Autodesk Inventor part; units mm, degrees
ref_plane "YZ Plane" through (0, 0, 0) normal (1, 0, 0) x (0, 1, 0)
ref_plane "XZ Plane" through (0, 0, 0) normal (0, 1, 0) x (-1, 0, 0)
ref_plane "XY Plane" through (0, 0, 0) normal (0, 0, 1) x (1, 0, 0)
sketch "草图1" plane through (0, 0, 0) normal (0, 1, 0) x (-1, 0, 0)
  circle A0 centre (-2.0908, 11.2121) radius 1.25
  line L0 (-5.7974, 4.2121) -> (1.6092, -1.1691) construction
  circle A1 centre (-11.3094, -1.4762) radius 1.25
  line L1 (0.7195, 14.068) -> (0.7195, -0.5227)
  line L2 (-4.7634, 3.4608) -> (-4.7634, 14.068)
  line L3 (-4.7634, 14.068) -> (0.7195, 14.068)
  line L4 (-13.1571, -5.0315) -> (0.7195, -0.5227)
  line L5 (-4.7634, 3.4608) -> (-14.8514, 0.183)
  line L6 (-14.8514, 0.183) -> (-13.1571, -5.0315)
  dimension "d12" = 2.5
extrude "拉伸1" add sketch "草图1" along normal blind 2
sketch "草图2" plane through (0, 2, 0) normal (0, 1, 0) x (1, 0, 0)
  circle A0 centre (11.3094, 1.4762) radius 1.25
  circle A1 centre (2.0908, -11.2121) radius 1.25
extrude "拉伸2" add sketch "草图2" against normal blind 2.1
sketch "草图3" plane through (11.3094, -0.1, -1.4762) normal (0, -1, 0) x (1, 0, 0)
  circle A0 centre (-9.2186, 12.6883) radius 1.25
  circle A1 centre (0, 0) radius 1.25
  circle A2 centre (-9.2186, 12.6883) radius 1.2
  circle A3 centre (0, 0) radius 1.2
  point P0 (-11.3094, 1.4762)
  dimension "d13" = 2.4
  dimension "d14" = 2.4
extrude "拉伸3" add sketch "草图3" along normal blind 15 contours A2 | A3
properties part number "鸦片"
Geometry check sheet. Reference: the model listing, model coordinates, mm. A direction names the side the tool comes from. Round coordinates to 2 decimals unless told otherwise and drop trailing zeros. Order: outer loops, then holes, each group sorted by start corner. A loop starts at its lowest first (then second) coordinate and runs counter-clockwise, first axis right, second up. Notation, with made-up numbers: M 58.25,80 L 92.25,80 A19 ccw 92.25,115 Z; hole C 43,-12.5 d11. An arc over 180 degrees is marked long. Answer in a Markdown table with one row per item. Add a question column.
Item 1: Depth check by flat-ended pin: pin 1 Ø4 at (x, y) = (13, -7.5) entering from +Z; pin 2 Ø8 at (y, z) = (-6, 7.5) entering from -X; pin 3 Ø4 at (x, y) = (7, -1.5) entering from +Z; pin 4 Ø1.5 at (y, z) = (-2, 6) entering from -X. Enter the tip coordinate at first touch or a pass-through.
Item 2: Sectioned sample at A-A, the plane x = 12. Enter the section's corners in (y, z).
Item 3: Set-up check for faces 1 (the face through (4.763, 1, 9)), 2 (the face through (11.049, -7.495, -0.305)), 3 (the face through (11, -15.1, -1)): record each of +Z, -Z, +X, -X, +Y, -Y from which the full face is reachable in a straight line by a thin tool's end or side.
Item 4: Sectioned sample at B-B, the plane y = -8.25. Enter the section's corners in (x, z), plus the area to 3 significant figures.
Item 5: Sectioned sample at C-C, the plane z = 2.75. Enter the section's corners in (x, y).
Item 6: Sectioned sample at D-D, the plane x = 1.5. Enter the section's corners in (y, z).
Item 7: Material ranges on L1, parallel to Y at x = 3, z = 9.25; L2, parallel to X at y = 1.25, z = 3.75; L3, parallel to Z at x = 11, y = -11.75, recorded low to high. Write a range as [from, to].
Filled in:
| question | item | result |
|---|---|---|
| 1 | pin 1 | stops at z = -0.28 |
| 1 | pin 2 | stops at x = 0.89 |
| 1 | pin 3 | stops at z = 3.16 |
| 1 | pin 4 | passes through |
| 2 | outline | M -15.1,-2.46 L -0.1,-2.46 L -0.1,-2.52 L 0,-2.52 L 0,-4.66 L 2,-4.66 L 2,1.11 L 0,1.11 L 0,-0.43 L -0.1,-0.43 L -0.1,-0.49 L -15.1,-0.49 Z |
| 3 | face 1 | +Z, +X, +Y, -Y |
| 3 | face 2 | -Y |
| 3 | face 3 | +Z, -Z, +X, -X, -Y |
| 4 | outline | C 2.09,11.21 d2.4; C 11.31,-1.48 d2.4 |
| 4 | area | 9.05 mm² |
| 5 | outline | M -0.72,0 L 6.95,0 L 6.95,2 L -0.72,2 Z |
| 6 | outline | M -15.1,10.17 L -0.1,10.17 L -0.1,10.11 L 0,10.11 L 0,-1.24 L 2,-1.24 L 2,14.07 L 0,14.07 L 0,12.31 L -0.1,12.31 L -0.1,12.26 L -15.1,12.26 Z |
| 7 | L1 | y = [0, 2] |
| 7 | L2 | x = [-0.72, 4.76] |
| 7 | L3 | z = [-2.64, -0.32] |
